Check sheet for the modelled part. Datum: model origin and axes. Units: mm. A direction names the side the tool comes from. Coordinates: 2 decimals unless noted, no trailing zeros. Use a Markdown table: item, result. Add a question column.
1) Tool access check on faces 4 (the flat face through (-21, 3.175, 2)), 5 (the cylindrical face through (0.081, 9.635, 1.565)), 6 (the flat face through (21, 3.175, 2)). Record the directions out of +Z, -Z, +X, -X, +Y, -Y that give a thin tool (end or side, any length) a straight path to the whole face; none if there is none.
2) Draft check along Y on faces 1 (the cylindrical face through (6.369, 4.067, 1.565)), 2 (the flat face through (-38.1, -5, 2)), 3 (the cylindrical face through (-0.515, 2.555, 1.565)). Enter one of: pulls with the +Y half, pulls with the -Y half, needs draft (parallel to the pull), parting line crosses it, or undercut.
3) Thickness scan on line 1 (Y direction, x = -2, z = 0.5); line 2 (X direction, y = 6, z = 1.8); line 3 (X direction, y = 4, z = 0.9). Record the ranges inside material, lowest first.
4) Go/stop test with a flat-tipped pin: P1, Ø1, axis at x = -17.5, z = 2, coming from the +Y side (3 decimals). Record where the tip stops, or that it passes through.
from build123d import *

# Parameters (mm, degrees)
F0_R     = 2.3749
F1_DEPTH = 3.175
F3_DEPTH = 25.4


with BuildPart() as f1:
    # F0 (on Top) → F1 (new body)
    with BuildSketch(Plane.XY):
        with BuildLine():
            Line((-38.1, -9.525), (38.1, -9.525))
            Line((38.1, -9.525), (38.1, -1.905))
            ThreePointArc((38.1, -1.905), (36.612102, 1.687102), (33.02, 3.175))
            Line((33.02, 3.175), (9.243306, 3.175))
            ThreePointArc((9.243306, 3.175), (6.333003, 4.091283), (4.472567, 6.509591))
            ThreePointArc((4.472567, 6.509591), (0, 9.635769), (-4.472567, 6.509591))
            ThreePointArc((-4.472567, 6.509591), (-6.333003, 4.091283), (-9.243306, 3.175))
            Line((-9.243306, 3.175), (-33.02, 3.175))
            ThreePointArc((-33.02, 3.175), (-36.612102, 1.687102), (-38.1, -1.905))
            Line((-38.1, -1.905), (-38.1, -9.525))
        make_face()
        with Locations((0, 4.873269)):
            Circle(F0_R, mode=Mode.SUBTRACT)
    extrude(amount=F1_DEPTH)

    # F2 (on face) → F3 (cut)
    with BuildSketch(Plane.XY.offset(3.175)):
        Polygon((-37.465, -9.525), (-38.1, -8.509), (-38.1, -14.148636), (38.1, -14.148636), (38.1, -8.509), (37.465, -9.525), (36.83, -8.509), (36.195, -9.525), (35.56, -8.509), (34.925, -9.525), (34.29, -8.509), (33.655, -9.525), (33.02, -8.509), (32.385, -9.525), (31.75, -8.509), (31.115, -9.525), (30.48, -8.509), (29.845, -9.525), (29.21, -8.509), (28.575, -9.525), (27.94, -8.509), (27.305, -9.525), (26.67, -8.509), (26.035, -9.525), (25.4, -8.509), (24.765, -9.525), (24.13, -8.509), (23.495, -9.525), (22.86, -8.509), (22.225, -9.525), (21.59, -8.509), (20.955, -9.525), (20.32, -8.509), (19.685, -9.525), (19.05, -8.509), (18.415, -9.525), (17.78, -8.509), (17.145, -9.525), (16.51, -8.509), (15.875, -9.525), (15.24, -8.509), (14.605, -9.525), (13.97, -8.509), (13.335, -9.525), (12.7, -8.509), (12.065, -9.525), (11.43, -8.509), (10.795, -9.525), (10.16, -8.509), (9.525, -9.525), (8.89, -8.509), (8.255, -9.525), (7.62, -8.509), (6.985, -9.525), (6.35, -8.509), (5.715, -9.525), (5.08, -8.509), (4.445, -9.525), (3.81, -8.509), (3.175, -9.525), (2.54, -8.509), (1.905, -9.525), (1.27, -8.509), (0.635, -9.525), (0, -8.509), (-0.635, -9.525), (-1.27, -8.509), (-1.905, -9.525), (-2.54, -8.509), (-3.175, -9.525), (-3.81, -8.509), (-4.445, -9.525), (-5.08, -8.509), (-5.715, -9.525), (-6.35, -8.509), (-6.985, -9.525), (-7.62, -8.509), (-8.255, -9.525), (-8.89, -8.509), (-9.525, -9.525), (-10.16, -8.509), (-10.795, -9.525), (-11.43, -8.509), (-12.065, -9.525), (-12.7, -8.509), (-13.335, -9.525), (-13.97, -8.509), (-14.605, -9.525), (-15.24, -8.509), (-15.875, -9.525), (-16.51, -8.509), (-17.145, -9.525), (-17.78, -8.509), (-18.415, -9.525), (-19.05, -8.509), (-19.685, -9.525), (-20.32, -8.509), (-20.955, -9.525), (-21.59, -8.509), (-22.225, -9.525), (-22.86, -8.509), (-23.495, -9.525), (-24.13, -8.509), (-24.765, -9.525), (-25.4, -8.509), (-26.035, -9.525), (-26.67, -8.509), (-27.305, -9.525), (-27.94, -8.509), (-28.575, -9.525), (-29.21, -8.509), (-29.845, -9.525), (-30.48, -8.509), (-31.115, -9.525), (-31.75, -8.509), (-32.385, -9.525), (-33.02, -8.509), (-33.655, -9.525), (-34.29, -8.509), (-34.925, -9.525), (-35.56, -8.509), (-36.195, -9.525), (-36.83, -8.509), align=None)
    extrude(amount=-F3_DEPTH, mode=Mode.SUBTRACT)


solid = f1.part
Solved:
| question | item | result |
|---|---|---|
| 1 | face 4 | +Z, -Z, -X, +Y |
| 1 | face 5 | +Z, -Z, +Y |
| 1 | face 6 | +Z, -Z, +X, +Y |
| 2 | face 1 | pulls with the +Y half |
| 2 | face 2 | needs draft |
| 2 | face 3 | undercut |
| 3 | line 1 | y = -9.37 to 3.59, 6.15 to 9.2 |
| 3 | line 2 | x = -4.69 to -2.09, 2.09 to 4.69 |
| 3 | line 3 | x = -6.47 to -2.21, 2.21 to 6.47 |
| 4 | P1 | stops at y = 3.175 |
